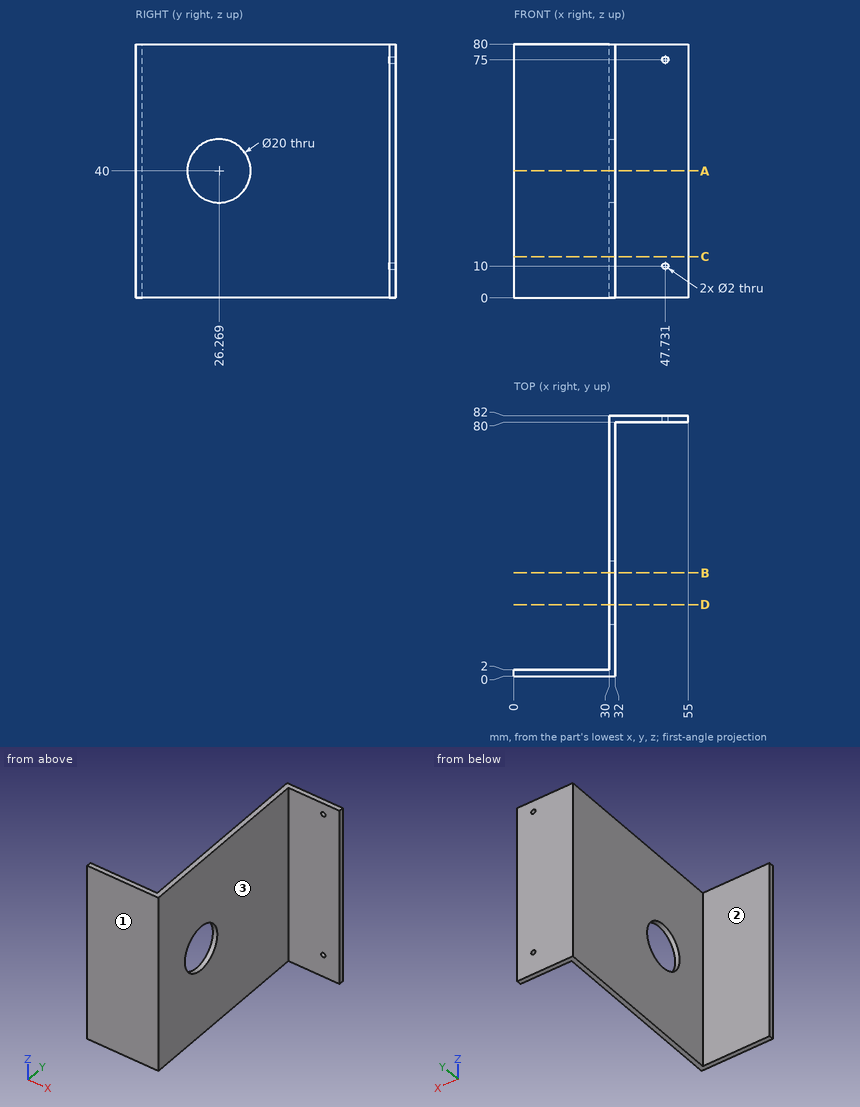
Could you check a few things on this drawing? It's one solid part, dimensions in mm from its lowest x, y, z. A direction names the side the tool comes from. Give positions to 0.01 mm unless a question says otherwise; leave off trailing zeros. Order: outer loops, then holes, each group sorted by start corner. A loop starts at its lowest first (then second) coordinate and runs counter-clockwise, first axis right, second up. Notation, with made-up numbers: (84.25, 59) -> (94.25, 59) arc R14 ccw to (94.25, 75) -> close; hole circle Ø6 at (80, 35). An arc over 180 degrees is marked (long way). Answer in a Markdown table with one row per item. Add a question column.
Item 1: I'm going to push flat-ended pins straight in: P1, Ø10, axis at y = 47.5, z = 22.5, coming from the -X side; P2, Ø1.5, axis at y = 47, z = 44, coming from the +X side; P3, Ø1.6, axis at x = 47.73, z = 75, coming from the +Y side; P4, Ø18.5, axis at x = 47, z = 31, coming from the -Y side. Where does each tip first touch, or does it pass through?
Item 2: Imagine slicing it at D-D (y = 22.5). List the corners of the cut face in (x, z) for me, and give its area (3 significant figures).
Item 3: For the marked faces 1, 2 and 3, which set-ups out of +Z, -Z, +X, -X, +Y, -Y let a thin tool reach every point of the face, with its end or its side?
Item 4: Imagine slicing it at B-B (y = 32.5). List the corners of the cut face in (x, z) for me.
Item 5: Imagine slicing it at A-A (z = 40). List the corners of the cut face in (x, y) for me, and give its area (3 significant figures).
Item 6: Imagine slicing it at C-C (z = 13). List the corners of the cut face in (x, y) for me, and give its area (3 significant figures).
Item 7: Please list where these lines run through material, in increasing order: probe 1 along X at (y, z) = (81, 10); probe 2 along Y at (x, z) = (34.5, 53.5); probe 3 along Y at (x, z) = (31.15, 40).
Result:
| question | item | result |
|---|---|---|
| 1 | P1 | x = 30 |
| 1 | P2 | x = 32 |
| 1 | P3 | through |
| 1 | P4 | y = 80 |
| 2 | outline | (30, 0) -> (32, 0) -> (32, 30.74) -> (30, 30.74) -> close; (30, 49.26) -> (32, 49.26) -> (32, 80) -> (30, 80) -> close |
| 2 | area | 123 mm2 |
| 3 | face 1 | +Z, -Z, +X, -X, -Y |
| 3 | face 2 | +Z, -Z, -X, +Y |
| 3 | face 3 | +Z, -Z, +X, -Y |
| 4 | outline | (30, 0) -> (32, 0) -> (32, 32.18) -> (30, 32.18) -> close; (30, 47.82) -> (32, 47.82) -> (32, 80) -> (30, 80) -> close |
| 5 | outline | (0, 0) -> (32, 0) -> (32, 16.27) -> (30, 16.27) -> (30, 2) -> (0, 2) -> close; (30, 36.27) -> (32, 36.27) -> (32, 80) -> (55, 80) -> (55, 82) -> (30, 82) -> close |
| 5 | area | 230 mm2 |
| 6 | outline | (0, 0) -> (32, 0) -> (32, 80) -> (55, 80) -> (55, 82) -> (30, 82) -> (30, 2) -> (0, 2) -> close |
| 6 | area | 270 mm2 |
| 7 | probe 1 | 30 to 46.73, 48.73 to 55 |
| 7 | probe 2 | 80 to 82 |
| 7 | probe 3 | 0 to 16.27, 36.27 to 82 |
